from build123d import *

# Parameters (mm, degrees)
SKETCH_1_W               = 168
SKETCH_1_H               = 168
EXTRUDE_1_DEPTH          = 5
CUT_EXTRUDE_1_DEPTH      = 6
SKETCH_5_R               = 51
CUT_EXTRUDE_4_DEPTH      = 6
SKETCH_6_R               = 1.65
CUT_EXTRUDE_5_DEPTH      = 6
PATTERN_CIRCULAR_2_COUNT = 12
SKETCH_7_R               = 2.65
CUT_EXTRUDE_6_DEPTH      = 6
PATTERN_CIRCULAR_3_COUNT = 4
FILLET_1_R               = 10
CUT_EXTRUDE_7_DEPTH      = 1
CUT_EXTRUDE_7_DEPTH_BACK = 6
FILLET_2_R               = 8
FILLET_3_R               = 5


with BuildPart() as part:
    # 草图1 → 凸台-拉伸1 (new body)
    with BuildSketch(Plane.XY):
        Rectangle(SKETCH_1_W, SKETCH_1_H)
    extrude(amount=EXTRUDE_1_DEPTH)

    # 草图2 → 切除-拉伸1 (cut, through all)
    with BuildSketch(Plane.XY.offset(5)):
        Polygon((64, 84), (84, 64), (84, 84), align=None)
        Polygon((64, -84), (84, -84), (84, -64), align=None)
        Polygon((-84, -64), (-84, -84), (-64, -84), align=None)
        Polygon((-64, 84), (-84, 84), (-84, 64), align=None)
    extrude(amount=-CUT_EXTRUDE_1_DEPTH, mode=Mode.SUBTRACT)

    # 草图5 → 切除-拉伸4 (cut, through all)
    with BuildSketch(Plane(origin=(0, 0, 0), x_dir=(-1, 0, 0), z_dir=(0, 0, -1))):
        Circle(SKETCH_5_R)
    extrude(amount=-CUT_EXTRUDE_4_DEPTH, mode=Mode.SUBTRACT)

    # 草图6 → 切除-拉伸5 (cut, through all)
    with BuildSketch(Plane(origin=(0, 0, 0), x_dir=(-1, 0, 0), z_dir=(0, 0, -1))):
        with Locations((-39.597979746, -39.597979746)):
            Circle(SKETCH_6_R)
    cut_extrude_5 = extrude(amount=-CUT_EXTRUDE_5_DEPTH, mode=Mode.SUBTRACT)

    # 阵列(圆周)2: 切除-拉伸5 ×12 about axis
    pattern_circular_2_axis = Axis((0, 0, 0), (0, 0, 1))
    for i in range(1, PATTERN_CIRCULAR_2_COUNT):
        add(cut_extrude_5.rotate(pattern_circular_2_axis, i * 360 / PATTERN_CIRCULAR_2_COUNT), mode=Mode.SUBTRACT)

    # 草图7 → 切除-拉伸6 (cut, through all)
    with BuildSketch(Plane(origin=(0, 0, 0), x_dir=(-1, 0, 0), z_dir=(0, 0, -1))):
        with Locations((74.353553391, 63.746951673)):
            Circle(SKETCH_7_R)
        with Locations((63.746951673, 74.353553391)):
            Circle(SKETCH_7_R)
    cut_extrude_6 = extrude(amount=-CUT_EXTRUDE_6_DEPTH, mode=Mode.SUBTRACT)

    # 阵列(圆周)3: 切除-拉伸6 ×4 about axis
    pattern_circular_3_axis = Axis((0, 0, 0), (0, 0, 1))
    for i in range(1, PATTERN_CIRCULAR_3_COUNT):
        add(cut_extrude_6.rotate(pattern_circular_3_axis, i * 360 / PATTERN_CIRCULAR_3_COUNT), mode=Mode.SUBTRACT)

    # 圆角1
    fillet_1_edges = [part.edges().sort_by_distance(p)[0] for p in [
        (-64, 84, 2.5),
        (-84, 64, 2.5),
        (-84, -64, 2.5),
        (-64, -84, 2.5),
        (64, -84, 2.5),
        (84, -64, 2.5),
        (64, 84, 2.5),
        (84, 64, 2.5),
    ]]
    fillet(fillet_1_edges, radius=FILLET_1_R)

    # 草图8 → 切除-拉伸7 (cut, two sides)
    with BuildSketch(Plane(origin=(0, 0, 0), x_dir=(-1, 0, 0), z_dir=(0, 0, -1))) as cut_extrude_7_sk:
        Polygon((-84, -52.887301628), (-84, 52.887301628), (-76.928932188, 45.816233816), (-76.928932188, -45.816233816), align=None)
        Polygon((-52.887301628, 84), (52.887301628, 84), (45.816233816, 76.928932188), (-45.816233816, 76.928932188), align=None)
        Polygon((84, 52.887301628), (76.928932188, 45.816233816), (76.928932188, -45.816233816), (84, -52.887301628), align=None)
        Polygon((52.887301628, -84), (-52.887301628, -84), (-45.816233816, -76.928932188), (45.816233816, -76.928932188), align=None)
    extrude(amount=CUT_EXTRUDE_7_DEPTH, mode=Mode.SUBTRACT)
    extrude(cut_extrude_7_sk.sketch, amount=-CUT_EXTRUDE_7_DEPTH_BACK, mode=Mode.SUBTRACT)

    # 圆角2
    fillet_2_edges = [part.edges().sort_by_distance(p)[0] for p in [
        (76.928932188, 45.816233816, 2.5),
        (76.928932188, -45.816233816, 2.5),
        (45.816233816, 76.928932188, 2.5),
        (-45.816233816, 76.928932188, 2.5),
        (-76.928932188, -45.816233816, 2.5),
        (-76.928932188, 45.816233816, 2.5),
        (-45.816233816, -76.928932188, 2.5),
        (45.816233816, -76.928932188, 2.5),
    ]]
    fillet(fillet_2_edges, radius=FILLET_2_R)

    # 圆角3
    fillet_3_edges = [part.edges().sort_by_distance(p)[0] for p in [
        (84, 52.887301628, 2.5),
        (84, -52.887301628, 2.5),
        (52.887301628, 84, 2.5),
        (-52.887301628, 84, 2.5),
        (-84, 52.887301628, 2.5),
        (-84, -52.887301628, 2.5),
        (-52.887301628, -84, 2.5),
        (52.887301628, -84, 2.5),
    ]]
    fillet(fillet_3_edges, radius=FILLET_3_R)


solid = part.part
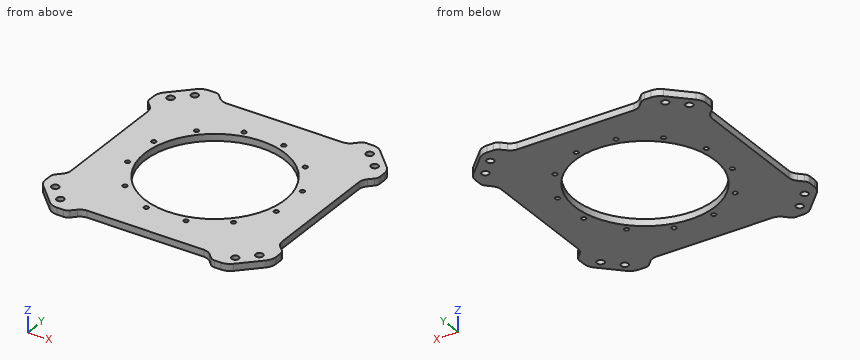
Design review of the part built by this model. Coordinates are the model's own, in mm. Round coordinates to 2 decimals unless told otherwise and drop trailing zeros. Write each loop counter-clockwise with the first axis right and the second up, starting at its lowest first coordinate (ties: lowest second). Pieces come first, ordered by that corner, then holes.
Item 1: For pin 1 Ø2 at (y, z) = (-13.5, 4) entering from -X; pin 2 Ø2.5 at (x, y) = (54.09, 14.49) entering from -Z; pin 3 Ø1.5 at (x, z) = (-7, 3) entering from +Y; pin 4 Ø1.5 at (x, z) = (16, 2.5) entering from -Y, all flat-tipped, find the tip position at first contact; note any pin that passes through.
Item 2: Consider section A-A on x = 0. Give the boundary of the cut face in (y, z), and give its area (3 significant figures).
Item 3: Consider section C-C on z = 3.15. Count the separate pieces of the cut face and the enclosed holes in it, and give its area (3 significant figures).
Item 4: Wall thickness on L1, parallel to Y at x = -2, z = 0.65; L2, parallel to Y at x = -64.5, z = 3.8; L3, parallel to X at y = 41, z = 3.35: over which ranges is each line inside the solid? List them lowest first.
Check values:
1. pin 1: stops at x = -76.93
1. pin 2: passes through
1. pin 3: stops at y = 76.93
1. pin 4: stops at y = -76.93
2. outline: (-76.93, 0) - (-51, 0) - (-51, 5) - (-76.93, 5) - close; (51, 0) - (76.93, 0) - (76.93, 5) - (51, 5) - close
2. area: 259 mm2
3. separate pieces: 1
3. enclosed holes: 21
3. area: 16,200 mm2
4. L1: y = -76.93 to -50.96, 50.96 to 76.93
4. L2: y = -82.86 to -76.89, -71.81 to 71.81, 76.89 to 82.86
4. L3: x = -76.93 to -40.47, -38.73 to -30.33, 30.33 to 38.73, 40.47 to 76.93
